Geometry: final body of the model. Coordinates: model frame, mm. A direction names the side the tool comes from. Give positions to 0.01 mm unless a question says otherwise; leave off trailing zeros. Order: outer loops, then holes, each group sorted by start corner. A loop starts at its lowest first (then second) coordinate and runs counter-clockwise, first axis right, second up. Notation, with made-up numbers: (-38, 10) - (-28, 10) arc R22 cw to (-28, 49) - close; hole circle Ø10 at (24, 86). An arc over 180 degrees is marked (long way). Write item = value, one per line. Start each with the question number.
from build123d import *

# Parameters (mm, degrees)
SKETCH_1_W        = 5
SKETCH_1_H        = 25
EXTRUDE_1_DEPTH   = 20
EXTRUDE_1_2_DEPTH = 20
SKETCH_2_W        = 65
SKETCH_2_H        = 25
EXTRUDE_2_DEPTH   = 5


with BuildPart() as part:
    # Sketch 1 → Extrude 1 (new body)
    with BuildSketch(Plane(origin=(0, 0, 0), x_dir=(1, 0, 0), z_dir=(0, 1, 0))):
        with Locations((30, 0)):
            Rectangle(SKETCH_1_W, SKETCH_1_H)
    extrude(amount=EXTRUDE_1_DEPTH)



with BuildPart() as body_2:
    # Sketch 1 → Extrude 1 2 (new body)
    with BuildSketch(Plane(origin=(0, 0, 0), x_dir=(1, 0, 0), z_dir=(0, 1, 0))):
        with Locations((-30, 0)):
            Rectangle(SKETCH_1_W, SKETCH_1_H)
    extrude(amount=EXTRUDE_1_2_DEPTH)


with BuildPart() as part_1:
    add(part.part)

    add(body_2.part)  # Extrude 2 merges body 2
    # Sketch 2 → Extrude 2 (add)
    with BuildSketch(Plane(origin=(0, 20, 0), x_dir=(1, 0, 0), z_dir=(0, 1, 0))):
        Rectangle(SKETCH_2_W, SKETCH_2_H)
    extrude(amount=EXTRUDE_2_DEPTH)


solid = part_1.part
Q1. Material intervals for line 1 along X through (y, z) = (19.5, 6.25); line 2 along Y through (x, z) = (19, -1.75), sorted ascending. Write a range as from..to.
Q2. Section C-C, the plane x = -18. Return the cut outline in (y, z).
Q3. Pull-direction query (X, two-part tool) for faces 3 (the flat face through (27.5, 10, 0)), 4 (the flat face through (30, 0, 0)), 5 (the flat face through (32.5, 12, 0)); classes: +X half, -X half, draft (parallel to the pull), parting line (faces both ways), or undercut.
Q4. Set-up query: faces 1 (the flat face through (0, 25, 0)), 2 (the flat face through (0, 20, 0)). Return all of +Z, -Z, +X, -X, +Y, -Y with unobstructed straight access to the full face (end or side cutting, diameter ignored); none if empty.
Q5. Contact query for flat-ended pins moving along their axis: pin 1 (7.5 mm diameter, centred on x = -3, z = -6, fed in from -Y); pin 2 (1.5 mm diameter, centred on x = -12.5, y = 19, fed in from -Z). Output: stop coordinate, or through.
Q6. Section A-A, the plane y = 16.25. Return the cut outline in (x, z), then the cut area to 3 significant figures.
Q7. Section B-B, the plane z = -5.75. Return the cut outline in (x, y).
The answers:
q1.line_1 = -32.5..-27.5, 27.5..32.5
q1.line_2 = 20..25
q2.outline = (20, -12.5) - (25, -12.5) - (25, 12.5) - (20, 12.5) - close
q3.face_3 = undercut
q3.face_4 = draft
q3.face_5 = +X half
q4.face_1 = +Z, -Z, +X, -X, +Y
q4.face_2 = +Z, -Z, -Y
q5.pin_1 = 20
q5.pin_2 = through
q6.outline = (-32.5, -12.5) - (-27.5, -12.5) - (-27.5, 12.5) - (-32.5, 12.5) - close; (27.5, -12.5) - (32.5, -12.5) - (32.5, 12.5) - (27.5, 12.5) - close
q6.area = 250 mm²
q7.outline = (-32.5, 0) - (-27.5, 0) - (-27.5, 20) - (27.5, 20) - (27.5, 0) - (32.5, 0) - (32.5, 25) - (-32.5, 25) - close
